```python
from build123d import *

# Parameters (mm, degrees)
SKETCH1_W                = 33.6
SKETCH1_H                = 26.1
BOSS_EXTRUDE1_DEPTH      = 13.75
BOSS_EXTRUDE2_DEPTH      = 2.32
BOSS_EXTRUDE2_DEPTH_BACK = 1.68
SKETCH2_W                = 4.26
SKETCH2_H                = 22
SKETCH3_W                = 2
SKETCH3_H                = 18
CUT_EXTRUDE1_DEPTH       = 28.284995877
CHAMFER1_SIZE            = 2
FILLET1_R                = 1


with BuildPart() as part:
    # Sketch1 → Boss-Extrude1 (new body)
    with BuildSketch(Plane(origin=(0, 0, 0), x_dir=(1, 0, 0), z_dir=(0, 1, 0))):
        Rectangle(SKETCH1_W, SKETCH1_H)
    extrude(amount=BOSS_EXTRUDE1_DEPTH)

    # Sketch2 → Boss-Extrude2 (add, two sides: drawn at the far end of the back side and taken through both)
    with BuildSketch(Plane(origin=(0, 0, 0), x_dir=(1, 0, 0), z_dir=(0, 1, 0)).offset(-BOSS_EXTRUDE2_DEPTH_BACK)):
        with Locations((18.93, 0)):
            Rectangle(SKETCH2_W, SKETCH2_H)
        with Locations((-18.93, 0)):
            Rectangle(SKETCH2_W, SKETCH2_H)
    extrude(amount=BOSS_EXTRUDE2_DEPTH + BOSS_EXTRUDE2_DEPTH_BACK)

    # Sketch3 → Cut-Extrude1 (cut, through all)
    with BuildSketch(Plane(origin=(0, 2.32, 0), x_dir=(1, 0, 0), z_dir=(0, 1, 0))):
        with Locations((18.06, 0)):
            Rectangle(SKETCH3_W, SKETCH3_H)
        with Locations((-18.06, 0)):
            Rectangle(SKETCH3_W, SKETCH3_H)
    extrude(amount=-CUT_EXTRUDE1_DEPTH, mode=Mode.SUBTRACT)

    # Chamfer1
    # the kernel refuses this chamfer: 2 mm, written as the material it adds along each edge
    with BuildSketch(Plane(origin=(16.8, 0, -11), x_dir=(-0.9996219169112968, 0.027495876610586365, 0), z_dir=(0, 0, 1))) as chamfer1_piece_1_section:
        Polygon((CHAMFER1_SIZE * 0.999621916911, CHAMFER1_SIZE * 0.0274958766106), (-CHAMFER1_SIZE * 0.0274958766106, CHAMFER1_SIZE * 0.999621916911), (0, 0), align=None)
    chamfer1_piece_1 = extrude(amount=22, mode=Mode.PRIVATE)
    chamfer1_piece_1 = split(chamfer1_piece_1, bisect_by=Plane(origin=(16.11862069, -1.68, 0), z_dir=(0, 1, 0)), keep=Keep.TOP, mode=Mode.PRIVATE)
    add(chamfer1_piece_1)
    with BuildSketch(Plane(origin=(-16.8, 0, 11), x_dir=(0.9996219169112968, 0.027495876610586365, 0), z_dir=(0, 0, -1))) as chamfer1_piece_2_section:
        Polygon((CHAMFER1_SIZE * 0.999621916911, CHAMFER1_SIZE * 0.0274958766106), (-CHAMFER1_SIZE * 0.0274958766106, CHAMFER1_SIZE * 0.999621916911), (0, 0), align=None)
    chamfer1_piece_2 = extrude(amount=22, mode=Mode.PRIVATE)
    chamfer1_piece_2 = split(chamfer1_piece_2, bisect_by=Plane(origin=(-16.11862069, -1.68, 0), z_dir=(0, 1, 0)), keep=Keep.TOP, mode=Mode.PRIVATE)
    add(chamfer1_piece_2)

    # Fillet1
    fillet1_edges = [part.edges().sort_by_distance(p)[0] for p in [
        (21.06, 0.32, 11),
        (21.06, 0.32, -11),
        (-21.06, 0.32, -11),
        (-21.06, 0.32, 11),
        (-16.8, 6.875, -13.05),
        (16.8, 6.875, -13.05),
        (16.8, 6.875, 13.05),
        (-16.8, 6.875, 13.05),
    ]]
    fillet(fillet1_edges, radius=FILLET1_R)


solid = part.part
```
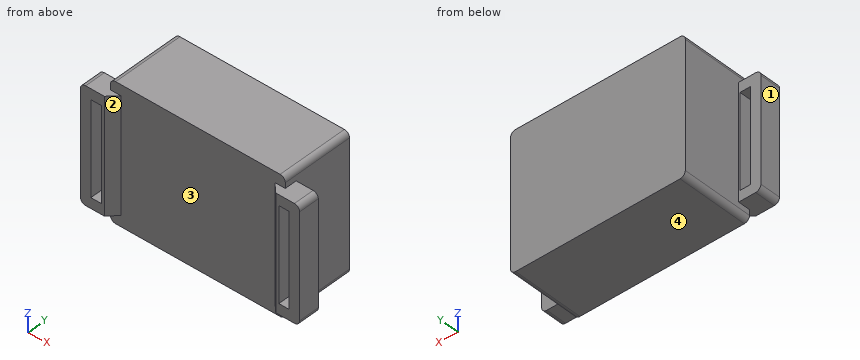
Part model, mm, in its own coordinate system. Face numbers are marked on the shaded views. Round coordinates to 2 decimals unless told otherwise and drop trailing zeros. Order: outer loops, then holes, each group sorted by start corner. A loop starts at its lowest first (then second) coordinate and runs counter-clockwise, first axis right, second up. Notation, with made-up numbers: M -30,-16.75 L 2,-16.75 A25 ccw 2,-2.75 Z; hole C 39,83 d4. An arc over 180 degrees is marked long. Put each result on its own line as item: value. Start each with the question number.
1. Drop flat-ended pins along their axis: pin 1 (2 mm diameter, centred on x = -17.5, y = 1.5, fed in from -Z); pin 2 (2 mm diameter, centred on x = 18.5, y = 0.5, fed in from -Z); pin 3 (2 mm diameter, centred on x = 18, y = 1, fed in from +Z). Give the stop position or say it passes through.
2. Slice it at C-C on y = 5.5. List the corners of the cut face in (x, z).
3. Drill centre lines: probe 1 along X at (y, z) = (1, -6.25); probe 2 along Z at (x, y) = (-18, -0.25); probe 3 along X at (y, z) = (8.25, -3.25). Where is each one in solid material? Low to high. Write a range as [from, to].
4. Slice it at D-D on x = -2.5. List the corners of the cut face in (y, z).
5. Two-plate mould, pull along X, no slides. Class the marked faces 1, 2, 3 and 4: +X half, -X half, draft (parallel to the pull), parting line (faces both ways), or undercut.
6. Slice it at A-A on y = -0.5. List the corners of the cut face in (x, z).
7. Slice it at B-B on z = -2. List the corners of the cut face in (x, y), then the cut area to 3 significant figures.
Findings:
1. pin 1: z = -12.76
1. pin 2: z = -11
1. pin 3: z = 11
2. outline: M -16.8,-12.05 A1 ccw -15.8,-13.05 L 15.8,-13.05 A1 ccw 16.8,-12.05 L 16.8,12.05 A1 ccw 15.8,13.05 L -15.8,13.05 A1 ccw -16.8,12.05 Z
3. probe 1: [-21.06, -19.06], [-17.06, 17.06], [19.06, 21.06]
3. probe 2: [-11, -9], [9, 11]
3. probe 3: [-16.8, 16.8]
4. outline: M 0,-13.05 L 13.75,-13.05 L 13.75,13.05 L 0,13.05 Z
5. face 1: -X half
5. face 2: undercut
5. face 3: undercut
5. face 4: draft
6. outline: M -21.06,-10 A1 ccw -20.06,-11 L -15.3,-11 L -15.3,11 L -20.06,11 A1 ccw -21.06,10 Z; M 15.3,-11 L 20.06,-11 A1 ccw 21.06,-10 L 21.06,10 A1 ccw 20.06,11 L 15.3,11 Z; hole M -19.06,-9 L -17.06,-9 L -17.06,9 L -19.06,9 Z; hole M 17.06,-9 L 19.06,-9 L 19.06,9 L 17.06,9 Z
7. outline: M -21.06,-1.68 L -19.06,-1.68 L -19.06,2.32 L -21.06,2.32 Z; M -17.06,-1.68 L -16.48,-1.68 L -14.8,0 L 14.8,0 L 16.48,-1.68 L 17.06,-1.68 L 17.06,2.32 L 16.8,2.32 L 16.8,13.75 L -16.8,13.75 L -16.8,2.32 L -17.06,2.32 Z; M 19.06,-1.68 L 21.06,-1.68 L 21.06,2.32 L 19.06,2.32 Z
7. area: 484 mm2
